Read the model definition and answer for the solid it produces. Units are mm, in the model's axes. Face numbers are marked on the shaded views. Round coordinates to 2 decimals unless told otherwise and drop trailing zeros. Write each loop counter-clockwise with the first axis right and the second up, starting at its lowest first coordinate (ties: lowest second). Pieces come first, ordered by that corner, then holes. Notation, with made-up numbers: (-2, 49) -> (43, 49) arc R27 cw to (43, 84) -> close; hole circle Ø8 at (-29, -33.75). An arc over 180 degrees is marked (long way). Return JSON: item names as keys, results as strings.
from build123d import *

# Parameters (mm, degrees)
F0_R      = 304.8
F1_DEPTH  = 6.35
F2_R      = 88.9
F2_R_2    = 85.725
F3_DEPTH  = 127
F4_DEPTH  = 25.4
F5_START  = 127
F2_R_3    = 139.7
F5_DEPTH  = 25.4
F6_START  = 152.4
F2_R_4    = 152.4
F6_DEPTH  = 25.4
F7_START  = 177.8
F7_DEPTH  = 25.4
F2_R_5    = 15.875
F8_DEPTH  = 25.4
F2_R_6    = 19.05
F9_DEPTH  = 38.1
F10_START = 38.1
F2_R_7    = 34.925
F10_DEPTH = 12.7


with BuildPart() as f1:
    # F0 (on Front) → F1 (new body)
    with BuildSketch(Plane.XZ):
        Circle(F0_R)
    extrude(amount=F1_DEPTH)

    # F2 (on face) → F3 (join)
    with BuildSketch(Plane.XZ.offset(6.35)):
        Circle(F2_R)
        Circle(F2_R_2, mode=Mode.SUBTRACT)
    extrude(amount=F3_DEPTH)

    # F2 (on face) → F4 (cut)
    with BuildSketch(Plane.XZ.offset(6.35)):
        Circle(F2_R_2)
    extrude(amount=-F4_DEPTH, mode=Mode.SUBTRACT)

    # F2 (on face) → F5 (join)
    with BuildSketch(Plane.XZ.offset(6.35).offset(F5_START)):
        Circle(F2_R_3)
        Circle(F2_R, mode=Mode.SUBTRACT)
        Circle(F2_R)
        Circle(F2_R_2, mode=Mode.SUBTRACT)
        Circle(F2_R_2)
    extrude(amount=F5_DEPTH)

    # F2 (on face) → F6 (join)
    with BuildSketch(Plane.XZ.offset(6.35).offset(F6_START)):
        Circle(F2_R_4)
        Circle(F2_R_3, mode=Mode.SUBTRACT)
        Circle(F2_R_3)
        Circle(F2_R, mode=Mode.SUBTRACT)
        Circle(F2_R)
        Circle(F2_R_2, mode=Mode.SUBTRACT)
        Circle(F2_R_2)
    extrude(amount=F6_DEPTH)

    # F2 (on face) → F7 (join)
    with BuildSketch(Plane.XZ.offset(6.35).offset(F7_START)):
        Circle(F2_R_3)
        Circle(F2_R, mode=Mode.SUBTRACT)
        Circle(F2_R)
        Circle(F2_R_2, mode=Mode.SUBTRACT)
        Circle(F2_R_2)
    extrude(amount=F7_DEPTH)

    # F2 (on face) → F8 (cut)
    with BuildSketch(Plane.XZ.offset(6.35)):
        with Locations((0, -247.65)):
            Circle(F2_R_5)
    extrude(amount=-F8_DEPTH, mode=Mode.SUBTRACT)

    # F2 (on face) → F9 (join)
    with BuildSketch(Plane.XZ.offset(6.35)):
        with Locations((0, -247.65)):
            Circle(F2_R_6)
        with Locations((0, -247.65)):
            Circle(F2_R_5, mode=Mode.SUBTRACT)
    extrude(amount=F9_DEPTH)

    # F2 (on face) → F10 (join)
    with BuildSketch(Plane.XZ.offset(6.35).offset(F10_START)):
        with Locations((0, -247.65)):
            Circle(F2_R_7)
        with Locations((0, -247.65)):
            Circle(F2_R_6, mode=Mode.SUBTRACT)
        with Locations((0, -247.65)):
            Circle(F2_R_6)
        with Locations((0, -247.65)):
            Circle(F2_R_5, mode=Mode.SUBTRACT)
        with Locations((0, -247.65)):
            Circle(F2_R_5)
    extrude(amount=F10_DEPTH)


solid = f1.part
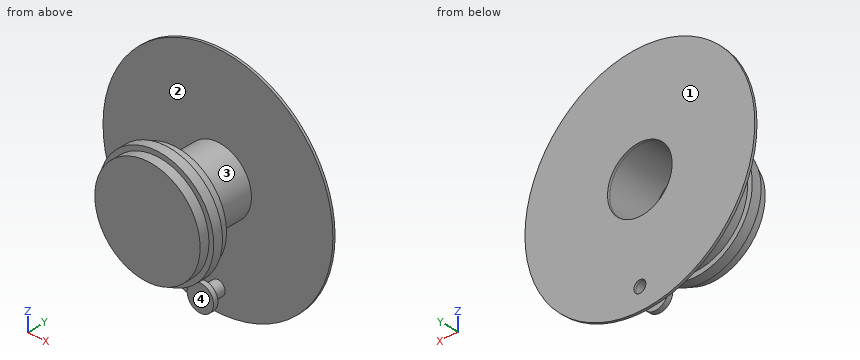
Item 1: For a pull along Y with two mould halves and no side action, classify the marked faces 1, 2, 3 and 4 as released by +Y, released by -Y, zero draft, split by the parting line, or undercut.
Worked answers:
{"face 1": "released by +Y", "face 2": "undercut", "face 3": "undercut", "face 4": "released by -Y"}
Item 2: Section A-A (z = 0) is taken. Give the vertices of the cut face in (x, y) (3 decimals).
Worked answers:
{"outline": "(-304.8, -6.35) -> (-88.9, -6.35) -> (-88.9, -133.35) -> (-139.7, -133.35) -> (-139.7, -158.75) -> (-152.4, -158.75) -> (-152.4, -184.15) -> (-139.7, -184.15) -> (-139.7, -209.55) -> (139.7, -209.55) -> (139.7, -184.15) -> (152.4, -184.15) -> (152.4, -158.75) -> (139.7, -158.75) -> (139.7, -133.35) -> (88.9, -133.35) -> (88.9, -6.35) -> (304.8, -6.35) -> (304.8, 0) -> (85.725, 0) -> (85.725, -133.35) -> (-85.725, -133.35) -> (-85.725, 0) -> (-304.8, 0) -> close"}
Item 3: Section D-D (y = -93.5) is taken. Give the vertices of the cut face in (x, z) (3 decimals).
Worked answers:
{"outline": "circle Ø177.8 at (0, 0); hole circle Ø171.45 at (0, 0)"}
Item 4: Section B-B (x = -103) is taken. Give the vertices of the cut face in (y, z).
Worked answers:
{"outline": "(-209.55, -94.38) -> (-184.15, -94.38) -> (-184.15, -112.32) -> (-158.75, -112.32) -> (-158.75, -94.38) -> (-133.35, -94.38) -> (-133.35, 94.38) -> (-158.75, 94.38) -> (-158.75, 112.32) -> (-184.15, 112.32) -> (-184.15, 94.38) -> (-209.55, 94.38) -> close; (-6.35, -286.87) -> (0, -286.87) -> (0, 286.87) -> (-6.35, 286.87) -> close"}
Item 5: Flat-ended cylindrical pins translate along their axes: pin 1 (2 mm diameter, centred on x = -242, z = -151, fed in from -Y); pin 2 (6 mm diameter, centred on y = -181.5, z = 116.5, fed in from +X); pin 3 (12 mm diameter, centred on x = 88.5, y = -38.5, fed in from +Z). Find the tip coordinate at first contact, or state that the pin passes through.
Worked answers:
{"pin 1": "stops at y = -6.35", "pin 2": "stops at x = 101.7", "pin 3": "stops at z = 33.12"}
Item 6: Straight lines are drawn through the part: L1, parallel to Z at x = 0, y = -2 (3 decimals); L2, parallel to Y at x = -59, z = -126; L3, parallel to X at y = -21, z = -247. For each, find the intervals that lie inside material, in ascending order. Write a range as [from, to].
Worked answers:
{"L1": "z = [-304.8, -263.525], [-231.775, -85.725], [85.725, 304.8]", "L2": "y = [-209.55, -133.35], [-6.35, 0]", "L3": "x = [-19.04, -15.86], [15.86, 19.04]"}
Item 7: Section C-C (y = -13.5) is taken. Give the vertices of the cut face in (x, z) (3 decimals).
Worked answers:
{"outline": "circle Ø177.8 at (0, 0); circle Ø38.1 at (0, -247.65); hole circle Ø171.45 at (0, 0); hole circle Ø31.75 at (0, -247.65)"}
